Geometry: see drawing. Coordinates: mm, zero at the bounding-box minimum. A direction names the side the tool comes from. Coordinates: 2 decimals unless noted, no trailing zeros. Loops run counter-clockwise (first coordinate to the right, second up) from the corner with the lowest first, then second, coordinate; pieces in that order, holes last. Notation, with made-up numbers: (34, 79) -> (70, 79) arc R23 cw to (70, 94) -> close; hole circle Ø2 at (81, 82). An arc over 180 degrees is marked (long way). One line per item, written item: value. Start each with the question number.
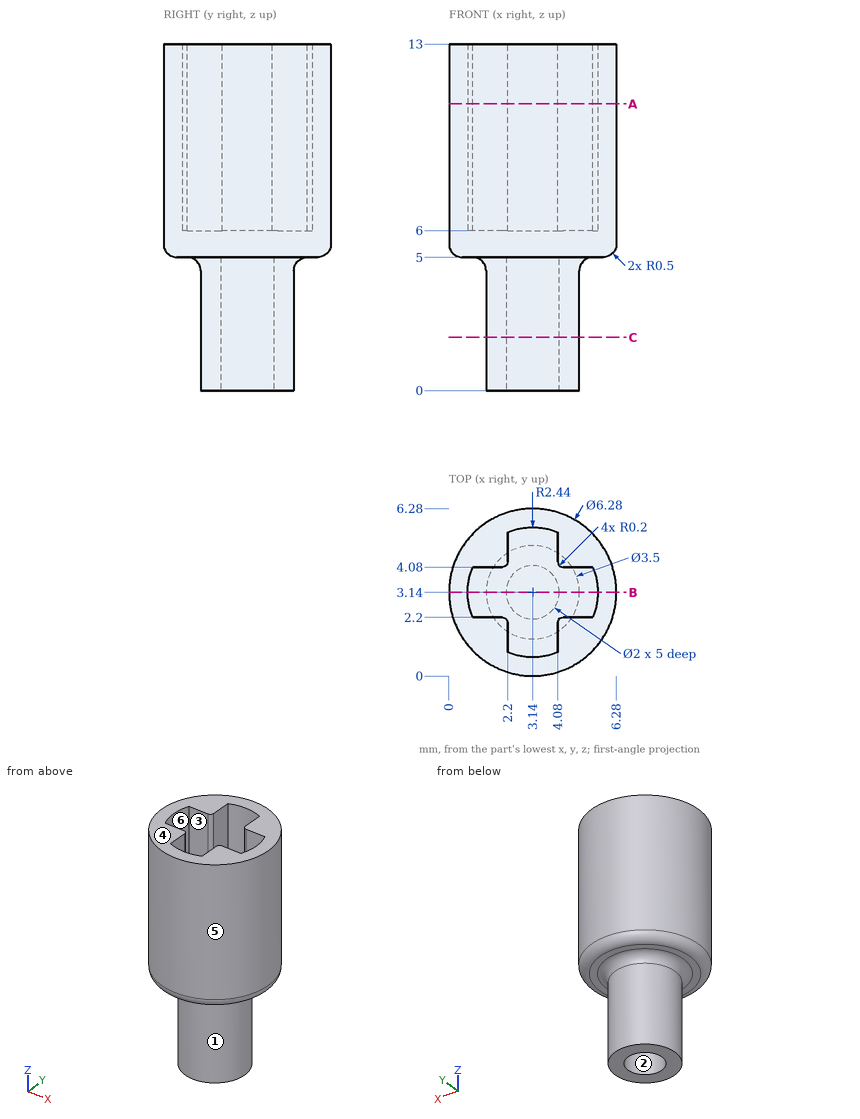
1. Set-up query: the marked faces 5 and 6. Return all of +Z, -Z, +X, -X, +Y, -Y with unobstructed straight access to the full face (end or side cutting, diameter ignored); none if empty.
2. Pin query (flat end, axial travel): pin 1 Ø1.2 at (x, z) = (5, 10) entering from -Y; pin 2 Ø2.5 at (x, y) = (3.14, 3.14) entering from -Z; pin 3 Ø0.9 at (y, z) = (4.5, 9.5) entering from +X; pin 4 Ø3 at (x, z) = (5.5, 9.5) entering from -Y. Return the tip coordinate at first contact, or that it passes through.
3. Line query: L1, parallel to Y at x = 3.14, z = 1.4; L2, parallel to Z at x = 5, y = 1.75; L3, parallel to Z at x = 4.5, y = 3.25. Output: solid intervals per line, ascending. Write a range as [from, to].
4. Section B-B on y = 3.14. Return the cut outline in (x, z).
5. Draft query along X for the marked faces 1, 2, 3 and 4. Return one class per face: released by +X, released by -X, zero draft, split by the parting line, or undercut.
6. Section C-C on z = 2. Return the cut outline in (x, y).
7. Section A-A on z = 10.75. Return the cut outline in (x, y), plus the area to 3 significant figures.
Checks:
1. face 5: +Z, -Z
1. face 6: +Z
2. pin 1: y = 0.26
2. pin 2: z = 0
2. pin 3: x = 6.15
2. pin 4: y = 0.12
3. L1: [1.39, 2.14], [4.14, 4.89]
3. L2: [5, 13]
3. L3: [0, 6]
4. outline: (0, 5.5) arc R0.5 ccw to (0.5, 5) -> (0.89, 5) arc R0.5 cw to (1.39, 4.5) -> (1.39, 0) -> (2.14, 0) -> (2.14, 5) -> (4.14, 5) -> (4.14, 0) -> (4.89, 0) -> (4.89, 4.5) arc R0.5 cw to (5.39, 5) -> (5.78, 5) arc R0.5 ccw to (6.28, 5.5) -> (6.28, 13) -> (5.58, 13) -> (5.58, 6) -> (0.7, 6) -> (0.7, 13) -> (0, 13) -> close
5. face 1: split by the parting line
5. face 2: undercut
5. face 3: undercut
5. face 4: zero draft
6. outline: circle Ø3.5 at (3.14, 3.14); hole circle Ø2 at (3.14, 3.14)
7. outline: circle Ø6.28 at (3.14, 3.14); hole (0.89, 2.2) -> (2, 2.2) arc R0.2 cw to (2.2, 2) -> (2.2, 0.89) arc R2.44 ccw to (4.08, 0.89) -> (4.08, 2) arc R0.2 cw to (4.28, 2.2) -> (5.39, 2.2) arc R2.44 ccw to (5.39, 4.08) -> (4.28, 4.08) arc R0.2 cw to (4.08, 4.28) -> (4.08, 5.39) arc R2.44 ccw to (2.2, 5.39) -> (2.2, 4.28) arc R0.2 cw to (2, 4.08) -> (0.89, 4.08) arc R2.44 ccw to start
7. area: 16.6 mm²
